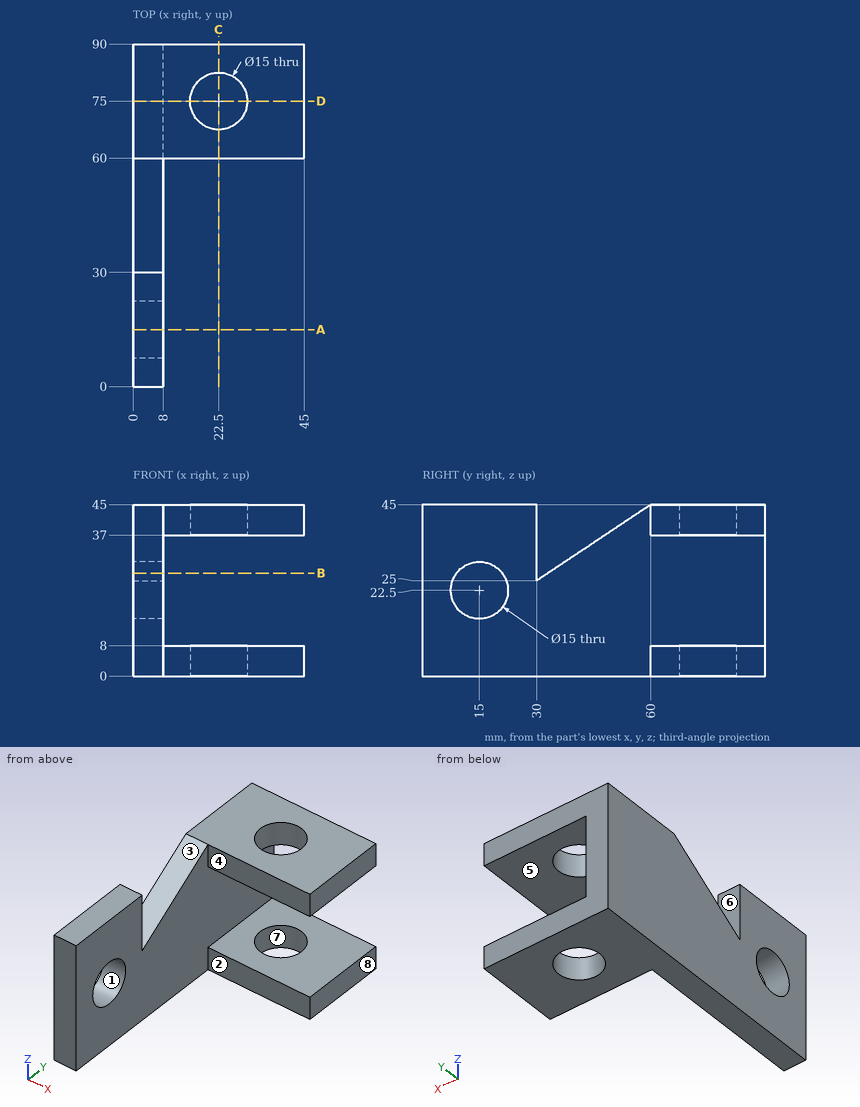
Geometry check sheet. Reference: drawing and pictorial views, mm from the part's lowest x, y, z. A direction names the side the tool comes from. Round coordinates to 2 decimals unless told otherwise and drop trailing zeros. Order: outer loops, then holes, each group sorted by start corner. A loop starts at its lowest first (then second) coordinate and runs counter-clockwise, first axis right, second up. Notation, with made-up numbers: M 84,3.5 L 111,3.5 A28 cw 111,29.5 Z; hole C -24,40 d10. An arc over 180 degrees is marked long. Write item = value, one per line.
Q1. Section check A-A (y = 15). Enter the section's corners in (x, z), plus the area to 3 significant figures.
Answer block:
outline = M 0,0 L 8,0 L 8,15 L 0,15 Z; M 0,30 L 8,30 L 8,45 L 0,45 Z
area = 240 mm^2
Q2. Section check C-C (x = 22.5). Enter the section's corners in (y, z).
Answer block:
outline = M 60,0 L 67.5,0 L 67.5,8 L 60,8 Z; M 60,37 L 67.5,37 L 67.5,45 L 60,45 Z; M 82.5,0 L 90,0 L 90,8 L 82.5,8 Z; M 82.5,37 L 90,37 L 90,45 L 82.5,45 Z
Q3. Scan lines: line 1 (Y direction, x = 22.5, z = 3.25); line 2 (Z direction, x = 14.5, y = 83.5); line 3 (Z direction, x = 3, y = 15). Record each from-to range of solid material in increasing order.
Answer block:
line_1 = 60 to 67.5, 82.5 to 90
line_2 = 0 to 8, 37 to 45
line_3 = 0 to 15, 30 to 45
Q4. Depth check by flat-ended pin: pin 1 Ø3 at (y, z) = (26, 27) entering from -X; pin 2 Ø2 at (y, z) = (15.5, 40) entering from +X; pin 3 Ø6.5 at (x, z) = (29, 39.5) entering from -Y; pin 4 Ø12 at (y, z) = (15, 22.5) entering from -X. Enter the tip coordinate at first touch or a pass-through.
Answer block:
pin_1 = 0
pin_2 = 8
pin_3 = 60
pin_4 = through
Q5. Section check D-D (y = 75). Enter the section's corners in (x, z).
Answer block:
outline = M 0,0 L 15,0 L 15,8 L 8,8 L 8,37 L 15,37 L 15,45 L 0,45 Z; M 30,0 L 45,0 L 45,8 L 30,8 Z; M 30,37 L 45,37 L 45,45 L 30,45 Z
Q6. Set-up check for the marked faces 4, 5, 6, 7 and 8: record each of +Z, -Z, +X, -X, +Y, -Y from which the full face is reachable in a straight line by a thin tool's end or side.
Answer block:
face_4 = +Z, -Z, +X, -Y
face_5 = +X, +Y, -Y
face_6 = +Z, +X, -X
face_7 = +Z, -Z
face_8 = +Z, -Z, +X, +Y, -Y
Q7. Section check B-B (z = 27). Enter the section's corners in (x, y), plus the area to 3 significant figures.
Answer block:
outline = M 0,0 L 8,0 L 8,9 L 0,9 Z; M 0,21 L 8,21 L 8,30 L 0,30 Z; M 0,33 L 8,33 L 8,90 L 0,90 Z
area = 600 mm^2
Q8. Release check for a two-part mould opening along Z. For the marked faces 1, 2 and 3 record: released by +Z, released by -Z, zero draft, split by the parting line, or undercut.
Answer block:
face_1 = undercut
face_2 = zero draft
face_3 = released by +Z
